from build123d import *

# Parameters (mm, degrees)
SKETCH1_R           = 12
SKETCH1_R_2         = 10
BOSS_EXTRUDE1_DEPTH = 4.5
SKETCH2_R           = 15
SKETCH2_R_2         = 11
BOSS_EXTRUDE2_DEPTH = 1
SCALE1_SCALE        = 1.013


with BuildPart() as part:
    # Sketch1 → Boss-Extrude1 (new body)
    with BuildSketch(Plane.XY):
        Circle(SKETCH1_R)
        Circle(SKETCH1_R_2, mode=Mode.SUBTRACT)
    extrude(amount=BOSS_EXTRUDE1_DEPTH)

    # Sketch2 → Boss-Extrude2 (add)
    with BuildSketch(Plane.XY.offset(4.5)):
        Circle(SKETCH2_R)
        Circle(SKETCH2_R_2, mode=Mode.SUBTRACT)
    extrude(amount=-BOSS_EXTRUDE2_DEPTH)


with BuildPart() as part_1:
    # Scale1: scaled about (0, 0, 2.758064516)
    add(part.part.scale(SCALE1_SCALE).moved(Location((0, 0, -0.035854839))))


solid = part_1.part
Geometry check sheet. Reference: the model listing, model coordinates, mm. Round coordinates to 2 decimals unless told otherwise and drop trailing zeros. Order: outer loops, then holes, each group sorted by start corner. A loop starts at its lowest first (then second) coordinate and runs counter-clockwise, first axis right, second up. Notation, with made-up numbers: M -30,63 L -13,63 A29 cw -13,101 Z; hole C -23,-19 d2. An arc over 180 degrees is marked long. Answer in a Markdown table with one row per item.
(1) Sectioned sample at C-C, the plane z = 4.15. Record the cut outline in (x, y) (3 decimals).
Responses:
| item | result |
|---|---|
| outline | C 0,0 d30.39; hole C 0,0 d20.26 |
(2) Sectioned sample at D-D, the plane z = 0.7. Record the cut outline in (x, y).
Responses:
| item | result |
|---|---|
| outline | C 0,0 d24.31; hole C 0,0 d20.26 |
(3) Draft check along X on faces 1 (the face through (5.45, 8.54, 2.21)), 2 (the face through (11.595, 3.651, 1.712)), 3 (the face through (-0.1, 12.5, 3.51)). Enter one of: released by +X, released by -X, zero draft, split by the parting line, or undercut.
Responses:
| item | result |
|---|---|
| face 1 | undercut |
| face 2 | split by the parting line |
| face 3 | zero draft |
(4) Go/stop test with flat-tipped pins: P1, Ø10, axis at x = -10.5, y = 9, coming from the -Z side; P2, Ø1.5, axis at x = -4.5, z = 0.5, coming from the -Y side; P3, Ø2, axis at y = -11, z = 1, coming from the -X side; P4, Ø1, axis at x = -4, z = 1, coming from the +Y side. Record where each tip stops, or that it passes through.
Responses:
| item | result |
|---|---|
| P1 | stops at z = -0.04 |
| P2 | stops at y = -11.56 |
| P3 | stops at x = -6.91 |
| P4 | stops at y = 11.64 |
(5) Scan lines: probe 1 along Y at (x, z) = (0, 2.1); probe 2 along Z at (x, y) = (10.5, 7); probe 3 along X at (y, z) = (4.5, 3.6). Record each from-to range of solid material in increasing order. Write a range as from..to.
Responses:
| item | result |
|---|---|
| probe 1 | y = -12.16..-10.13, 10.13..12.16 |
| probe 2 | z = 3.51..4.52 |
| probe 3 | x = -14.51..-9.08, 9.08..14.51 |
(6) Sectioned sample at A-A, the plane x = 0. Record the cut outline in (y, z) (3 decimals).
Responses:
| item | result |
|---|---|
| outline | M -15.195,3.51 L -12.156,3.51 L -12.156,-0.036 L -10.13,-0.036 L -10.13,4.523 L -15.195,4.523 Z; M 10.13,-0.036 L 12.156,-0.036 L 12.156,3.51 L 15.195,3.51 L 15.195,4.523 L 10.13,4.523 Z |
